```python
from build123d import *

# Parameters (mm, degrees)
F1_DEPTH = 63.5
F2_DEPTH = 25.4
F3_DEPTH = 25.4
F4_DEPTH = 7.9375
F6_R     = 5.08
F7_R     = 5.08


with BuildPart() as f1:
    # F0 (on Front) → F1 (new body, symmetric)
    with BuildSketch(Plane.XZ):
        Polygon((-41.275, 9.525), (-41.275, -9.525), (41.275, -9.525), (41.275, 9.525), (22.225, 9.525), align=None)
    extrude(amount=F1_DEPTH, both=True)

    # F0 (on Front) → F2 (join, symmetric)
    with BuildSketch(Plane.XZ):
        with BuildLine():
            Line((22.225, 9.525), (41.275, 9.525))
            Line((41.275, 9.525), (41.275, 27.32094))
            ThreePointArc((41.275, 27.32094), (47.109768, 39.617662), (60.325, 42.8752))
            Line((60.325, 42.8752), (60.325, 62.001544))
            add(Edge.make_bspline(
                [(60.325, 62.001544), (57.988427, 62.097884), (55.662261, 62.10827), (53.349908, 62.038586)],
                knots=[1.216171, 1.216171, 1.216171, 1.216171, 6.730793, 6.730793, 6.730793, 6.730793], degree=3))
            ThreePointArc((53.349908, 62.038586), (31.145444, 50.634428), (22.225, 27.32094))
            Line((22.225, 27.32094), (22.225, 9.525))
        make_face()
    extrude(amount=F2_DEPTH, both=True)

    # F0 (on Front) → F3 (join, symmetric)
    with BuildSketch(Plane.XZ):
        with BuildLine():
            add(Edge.make_bspline(
                [(61.872375, 61.9252), (61.356101, 61.954871), (60.840298, 61.980297), (60.325, 62.001544)],
                knots=[0, 0, 0, 0, 1.216171, 1.216171, 1.216171, 1.216171], degree=3))
            Line((60.325, 62.001544), (60.325, 42.8752))
            Line((60.325, 42.8752), (85.725, 42.8752))
            Line((85.725, 42.8752), (85.725, 61.9252))
            Line((85.725, 61.9252), (61.872375, 61.9252))
        make_face()
    extrude(amount=F3_DEPTH, both=True)

    # F0 (on Front) → F4 (join, symmetric)
    with BuildSketch(Plane.XZ):
        with BuildLine():
            add(Edge.make_bspline(
                [(53.349908, 62.038586), (7.6601, 60.6617), (-32.637096, 28.024181), (-41.275, 9.525)],
                knots=[6.730793, 6.730793, 6.730793, 6.730793, 115.69426, 115.69426, 115.69426, 115.69426], degree=3))
            Line((-41.275, 9.525), (22.225, 9.525))
            Line((22.225, 9.525), (22.225, 27.32094))
            ThreePointArc((22.225, 27.32094), (31.145444, 50.634428), (53.349908, 62.038586))
        make_face()
    extrude(amount=F4_DEPTH, both=True)

    # F0 (on Front) → F5 (revolve)
    with BuildSketch(Plane.XZ):
        Polygon((85.725, 61.9252), (85.725, 42.8752), (85.725, 38.1), (111.125, 38.1), (111.125, 66.675), (85.725, 66.675), align=None)
    revolve(axis=Axis((85.725, 0, 52.3875), (0, 0, 1)))

    # F6
    f6_edges = [f1.edges().sort_by_distance(p)[0] for p in [
        (-41.275, 63.5, 0),
        (41.275, 63.5, 0),
        (-41.275, -63.5, 0),
    ]]
    fillet(f6_edges, radius=F6_R)

    # F7
    f7_edges = [f1.edges().sort_by_distance(p)[0] for p in [
        (41.275, -63.5, 0),
    ]]
    fillet(f7_edges, radius=F7_R)


solid = f1.part
```
Check sheet for the modelled part. Datum: model origin and axes. Units: mm. A direction names the side the tool comes from. Give positions to 0.01 mm unless a question says otherwise; leave off trailing zeros. Write each loop counter-clockwise with the first axis right and the second up, starting at its lowest first coordinate (ties: lowest second). Pieces come first, ordered by that corner, then holes.
Item 1: Access from +Z, -Z, +X, -X, +Y, -Y to the whole of each face (thin tool, end or side, straight path). Record for faces 1 (the face through (68, -21, 61.925)), 2 (the face through (5, -7.938, 30)), 3 (the face through (86, 0, 38.1)), 4 (the face through (22.225, 17, 19)), 5 (the face through (46, -25.4, 42)).
Item 2: Gauge pin test, flat ends, axial feed: pin 1 (16 mm diameter, centred on x = 69, z = 23, fed in from -Y); pin 2 (2 mm diameter, centred on x = 11.5, y = -3, fed in from +Z); pin 3 (6 mm diameter, centred on x = 73.5, y = -5, fed in from -Z); pin 4 (1 mm diameter, centred on x = -4.5, z = 41.5, fed in from +Y). Record the tip position at first contact, or that the pin passes through.
Item 3: Scan lines: L1, parallel to Y at x = 9.5, z = 50.5; L2, parallel to Z at x = 4, y = -56 (3 decimals); L3, parallel to Z at x = 74.5, y = 25. Record each from-to range of solid material in increasing order.
Item 4: Draft check along X on faces 6 (the face through (41.275, -1, 5)), 7 (the face through (-39.8, 62, -0.1)), 8 (the face through (65, 19, 42.875)). Enter one of: released by +X, released by -X, zero draft, split by the parting line, or undercut.
Item 5: Cross-section at B-B (y = -43). Enter the section's corners in (x, z) (3 decimals), and give its area (3 significant figures).
Item 6: Cross-section at A-A (z = -4). Enter the section's corners in (x, y) (3 decimals), and give its area (3 significant figures).
Item 7: Cross-section at C-C (x = 96). Enter the section's corners in (y, z) (3 decimals).
Report:
1. face 1: +Z, -Y
1. face 2: +Z, -X, -Y
1. face 3: -Z, +X, +Y, -Y
1. face 4: +Z, -X, +Y
1. face 5: +Z, +X, -X, -Y
2. pin 1: passes through
2. pin 2: stops at z = 52.81
2. pin 3: stops at z = 38.1
2. pin 4: stops at y = 7.94
3. L1: y = -7.94 to 7.94
3. L2: z = -9.525 to 9.525
3. L3: z = 42.88 to 61.93
4. face 6: released by +X
4. face 7: released by -X
4. face 8: undercut
5. outline: (-41.275, -9.525) - (41.275, -9.525) - (41.275, 9.525) - (-41.275, 9.525) - close
5. area: 1,570 mm2
6. outline: (-41.275, -58.42) arc R5.08 ccw to (-36.195, -63.5) - (36.195, -63.5) arc R5.08 ccw to (41.275, -58.42) - (41.275, 58.42) arc R5.08 ccw to (36.195, 63.5) - (-36.195, 63.5) arc R5.08 ccw to (-41.275, 58.42) - close
6. area: 10,500 mm2
7. outline: (-23.229, 38.1) - (23.229, 38.1) - (23.229, 66.675) - (-23.229, 66.675) - close
